Build history of the part. All positions in model axes, mm. A direction names the side the tool comes from. Round coordinates to 2 decimals unless told otherwise and drop trailing zeros. Loops run counter-clockwise (first coordinate to the right, second up) from the corner with the lowest first, then second, coordinate; pieces in that order, holes last. Notation, with made-up numbers: M 29.5,-8.75 L 50.5,-8.75 A17 ccw 50.5,3.25 Z; hole C -2.5,52.25 d1. An arc over 180 degrees is marked long. Use one line per item in the form item = value. Start each with the question number.
```python
from build123d import *

# Parameters (mm, degrees)
SKETCH1_W           = 31.75
SKETCH1_H           = 38.1
BOSS_EXTRUDE1_DEPTH = 6.35
SKETCH2_R           = 0.95
CUT_EXTRUDE1_DEPTH  = 26.597668351
SKETCH3_W           = 15
SKETCH3_H           = 5.08
CUT_EXTRUDE2_DEPTH  = 26.597668351
SKETCH4_W           = 31.75
SKETCH4_H           = 38.1
SKETCH4_W_2         = 26.416
SKETCH4_H_2         = 32.766
CUT_EXTRUDE3_DEPTH  = 3.175
FILLET1_R           = 3.175


with BuildPart() as part:
    # Sketch1 → Boss-Extrude1 (new body)
    with BuildSketch(Plane(origin=(0, 0, 0), x_dir=(1, 0, 0), z_dir=(0, 1, 0))):
        Rectangle(SKETCH1_W, SKETCH1_H)
    extrude(amount=BOSS_EXTRUDE1_DEPTH)

    # Sketch2 → Cut-Extrude1 (cut, through all)
    with BuildSketch(Plane(origin=(0, 6.35, 0), x_dir=(1, 0, 0), z_dir=(0, 1, 0))):
        with Locations(Location((-6.985, 2.54, 0), (0, 0, 270))):
            Circle(SKETCH2_R)
        with Locations(Location((6.985, 2.54, 0), (0, 0, 270))):
            Circle(SKETCH2_R)
        with Locations(Location((-6.985, 12.7, 0), (0, 0, 270))):
            Circle(SKETCH2_R)
        with Locations(Location((6.985, 12.7, 0), (0, 0, 270))):
            Circle(SKETCH2_R)
    extrude(amount=-CUT_EXTRUDE1_DEPTH, mode=Mode.SUBTRACT)

    # Sketch3 → Cut-Extrude2 (cut, through all)
    with BuildSketch(Plane(origin=(0, 6.35, 0), x_dir=(1, 0, 0), z_dir=(0, 1, 0))):
        with Locations((0, -10.16)):
            Rectangle(SKETCH3_W, SKETCH3_H)
    extrude(amount=-CUT_EXTRUDE2_DEPTH, mode=Mode.SUBTRACT)

    # Sketch4 → Cut-Extrude3 (cut)
    with BuildSketch(Plane(origin=(0, 6.35, 0), x_dir=(1, 0, 0), z_dir=(0, 1, 0))):
        Rectangle(SKETCH4_W, SKETCH4_H)
        Rectangle(SKETCH4_W_2, SKETCH4_H_2, mode=Mode.SUBTRACT)
    extrude(amount=-CUT_EXTRUDE3_DEPTH, mode=Mode.SUBTRACT)

    # Fillet1
    fillet1_edges = [part.edges().sort_by_distance(p)[0] for p in [
        (15.875, 1.5875, 19.05),
        (-15.875, 1.5875, 19.05),
        (-15.875, 1.5875, -19.05),
        (15.875, 1.5875, -19.05),
    ]]
    fillet(fillet1_edges, radius=FILLET1_R)


solid = part.part
```
Q1. Wall check: probe 1 along X at (y, z) = (5, -12.7) (3 decimals); probe 2 along Z at (x, y) = (0, 0.5); probe 3 along X at (y, z) = (2.25, -2.54) (3 decimals). Give the ranges that are in metal, low to high.
Q2. Saw through at C-C (x = -11.5). Give the cut face in (y, z) (3 decimals).
Q3. Saw through at A-A (x = 2.5). Give the cut face in (y, z) (3 decimals).
Q4. Pull direction X, two halves, no side cores. Call faces 1 (the face through (0, 3, 7.62)), 2 (the face through (-13.208, 5, 0)), 3 (the face through (0, 3, 12.7)), 4 (the face through (0, 2, -19.05)): pulls with the +X half, pulls with the -X half, needs draft (parallel to the pull), parting line crosses it, or undercut.
Q5. Drop flat-ended pins along their axis: P1, Ø1.6, axis at y = 5.5, z = 5, coming from the -X side; P2, Ø1.6, axis at x = -6.5, y = 5.5, coming from the +Z side. Give the stop position or say it passes through.
Q6. Saw through at B-B (z = -12.7). Give the cut face in (x, y) (3 decimals), and give its area (3 significant figures).
Q7. Tool access for faces 5 (the face through (0, 5, 16.383)), 6 (the face through (13.208, 5, 0)), 7 (the face through (-14, 3.175, 0)): list every direction of +Z, -Z, +X, -X, +Y, -Y with a clear straight run to the whole face (end or side of a thin tool).
Q8. Saw through at D-D (y = 5.25). Give the cut face in (x, z) (3 decimals), and give its area (3 significant figures).
Filled in:
q1.probe_1 = -13.208 to -7.935, -6.035 to 6.035, 7.935 to 13.208
q1.probe_2 = -19.05 to 7.62, 12.7 to 19.05
q1.probe_3 = -15.875 to -7.935, -6.035 to 6.035, 7.935 to 15.875
q2.outline = M 0,-19.05 L 3.175,-19.05 L 3.175,-16.383 L 6.35,-16.383 L 6.35,16.383 L 3.175,16.383 L 3.175,19.05 L 0,19.05 Z
q3.outline = M 0,-19.05 L 3.175,-19.05 L 3.175,-16.383 L 6.35,-16.383 L 6.35,7.62 L 0,7.62 Z; M 0,12.7 L 6.35,12.7 L 6.35,16.383 L 3.175,16.383 L 3.175,19.05 L 0,19.05 Z
q4.face_1 = undercut
q4.face_2 = pulls with the -X half
q4.face_3 = undercut
q4.face_4 = needs draft
q5.P1 = -13.21
q5.P2 = 16.38
q6.outline = M -15.875,0 L -7.935,0 L -7.935,6.35 L -13.208,6.35 L -13.208,3.175 L -15.875,3.175 Z; M -6.035,0 L 6.035,0 L 6.035,6.35 L -6.035,6.35 Z; M 7.935,0 L 15.875,0 L 15.875,3.175 L 13.208,3.175 L 13.208,6.35 L 7.935,6.35 Z
q6.area = 161 mm²
q7.face_5 = +Z, +X, -X, +Y
q7.face_6 = +Z, -Z, +X, +Y
q7.face_7 = +Y
q8.outline = M -13.208,-16.383 L 13.208,-16.383 L 13.208,16.383 L -13.208,16.383 Z; hole C -6.985,-12.7 d1.9; hole C -6.985,-2.54 d1.9; hole M -7.5,7.62 L 7.5,7.62 L 7.5,12.7 L -7.5,12.7 Z; hole C 6.985,-12.7 d1.9; hole C 6.985,-2.54 d1.9
q8.area = 778 mm²
